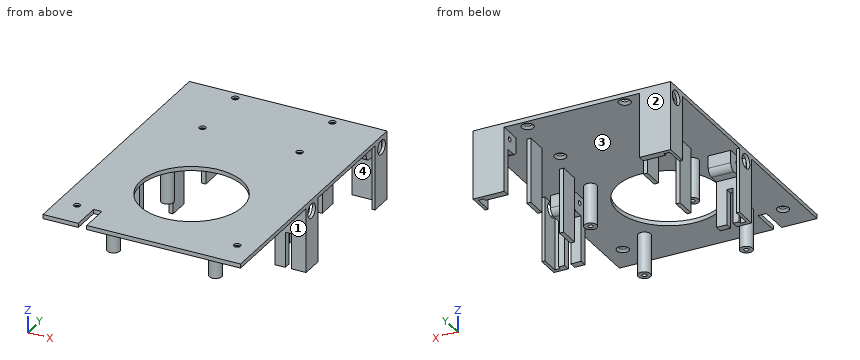
```python
from build123d import *

# Parameters (mm, degrees)
SKETCH1_W                                 = 95
SKETCH1_H                                 = 134
BOSS_EXTRUDE1_DEPTH                       = 2
CSK_FOR_4_FLAT_HEAD_MACHINE_SCREW_2_COUNT = 2
CSK_FOR_4_FLAT_HEAD_MACHINE_SCREW_2_PITCH = 46.7
CSK_FOR_4_FLAT_HEAD_MACHINE_SCREW_3_COUNT = 2
CSK_FOR_4_FLAT_HEAD_MACHINE_SCREW_3_PITCH = 55.505765466
CSK_FOR_4_FLAT_HEAD_MACHINE_SCREW_4_COUNT = 2
CSK_FOR_4_FLAT_HEAD_MACHINE_SCREW_4_PITCH = 30
CSK_FOR_4_FLAT_HEAD_MACHINE_SCREW_5_COUNT = 2
CSK_FOR_4_FLAT_HEAD_MACHINE_SCREW_5_PITCH = 116.985137945
CSK_FOR_4_FLAT_HEAD_MACHINE_SCREW_6_COUNT = 2
CSK_FOR_4_FLAT_HEAD_MACHINE_SCREW_6_PITCH = 131.458824352
SKETCH13_R                                = 24.6
CUT_EXTRUDE2_DEPTH                        = 165.271117364
SKETCH14_R                                = 3
BOSS_EXTRUDE4_DEPTH                       = 19.3
SKETCH15_R                                = 1.15
CUT_EXTRUDE3_DEPTH                        = 15
SKETCH16_W                                = 4
SKETCH16_H                                = 14
CUT_EXTRUDE4_DEPTH                        = 166.388905311
SKETCH17_W                                = 15
SKETCH17_H                                = 11
BOSS_EXTRUDE5_DEPTH                       = 31
SKETCH18_W                                = 2.7
SKETCH18_H                                = 70
CUT_EXTRUDE5_DEPTH                        = 31
SKETCH19_W                                = 14.3
SKETCH19_H                                = 67
CUT_EXTRUDE6_DEPTH                        = 22
FILLET5_R                                 = 3
FILLET6_R                                 = 3
FILLET7_R                                 = 3
FILLET8_R                                 = 3
SKETCH20_W                                = 2
SKETCH20_H                                = 10
BOSS_EXTRUDE6_DEPTH                       = 31
CUT_EXTRUDE7_DEPTH                        = 165.807888161
CUT_EXTRUDE7_DEPTH_BACK                   = 165.807888161
SKETCH22_R                                = 1.15
SKETCH23_R                                = 3.5
CUT_EXTRUDE8_DEPTH                        = 1.5
CUT_EXTRUDE9_START                        = -1.5
SKETCH24_R                                = 3.5
CUT_EXTRUDE9_DEPTH                        = 1.5
SKETCH25_W                                = 3
SKETCH25_H                                = 3.5
CUT_EXTRUDE10_DEPTH                       = 17


with BuildPart() as part:
    # Sketch1 → Boss-Extrude1 (new body)
    with BuildSketch(Plane.XY):
        with Locations((47.5, 67)):
            Rectangle(SKETCH1_W, SKETCH1_H)
    extrude(amount=BOSS_EXTRUDE1_DEPTH)

    # Sketch8 → CSK for #4 Flat Head Machine Screw (100)2 (revolve, cut)
    with BuildSketch(Plane(origin=(70.85, 130, 0), x_dir=(0, 1, 0), z_dir=(1, 0, 0))):
        Polygon((0, 0), (0, 2), (1.63195, 2), (1.63195, 1.028358553), (2.8575, 0), align=None)
    csk_for_4_flat_head_machine_screw_100 = revolve(axis=Axis((70.85, 130, -6.35), (0, 0, 1)), mode=Mode.SUBTRACT)

    # CSK for _4 Flat Head Machine Screw _ 2: CSK for #4 Flat Head Machine Screw (100)2 ×2
    with Locations(*[(-i * CSK_FOR_4_FLAT_HEAD_MACHINE_SCREW_2_PITCH, 0, 0) for i in range(1, CSK_FOR_4_FLAT_HEAD_MACHINE_SCREW_2_COUNT)]):
        add(csk_for_4_flat_head_machine_screw_100, mode=Mode.SUBTRACT)

    # CSK for _4 Flat Head Machine Screw _ 3: CSK for #4 Flat Head Machine Screw (100)2 ×2
    with Locations(*[Vector(-0.8413540396691381, -0.540484393791738, 0) * (i * CSK_FOR_4_FLAT_HEAD_MACHINE_SCREW_3_PITCH) for i in range(1, CSK_FOR_4_FLAT_HEAD_MACHINE_SCREW_3_COUNT)]):
        add(csk_for_4_flat_head_machine_screw_100, mode=Mode.SUBTRACT)

    # CSK for _4 Flat Head Machine Screw _ 4: CSK for #4 Flat Head Machine Screw (100)2 ×2
    with Locations(*[(0, -i * CSK_FOR_4_FLAT_HEAD_MACHINE_SCREW_4_PITCH, 0) for i in range(1, CSK_FOR_4_FLAT_HEAD_MACHINE_SCREW_4_COUNT)]):
        add(csk_for_4_flat_head_machine_screw_100, mode=Mode.SUBTRACT)

    # CSK for _4 Flat Head Machine Screw _ 5: CSK for #4 Flat Head Machine Screw (100)2 ×2
    with Locations(*[Vector(0.12950362982970207, -0.991578947870986, 0) * (i * CSK_FOR_4_FLAT_HEAD_MACHINE_SCREW_5_PITCH) for i in range(1, CSK_FOR_4_FLAT_HEAD_MACHINE_SCREW_5_COUNT)]):
        add(csk_for_4_flat_head_machine_screw_100, mode=Mode.SUBTRACT)

    # CSK for _4 Flat Head Machine Screw _ 6: CSK for #4 Flat Head Machine Screw (100)2 ×2
    with Locations(*[Vector(-0.47048952632046626, -0.8824055788710445, 0) * (i * CSK_FOR_4_FLAT_HEAD_MACHINE_SCREW_6_PITCH) for i in range(1, CSK_FOR_4_FLAT_HEAD_MACHINE_SCREW_6_COUNT)]):
        add(csk_for_4_flat_head_machine_screw_100, mode=Mode.SUBTRACT)

    # Sketch13 → Cut-Extrude2 (cut, through all)
    with BuildSketch(Plane(origin=(0, 0, 0), x_dir=(-1, 0, 0), z_dir=(0, 0, -1))):
        with Locations((-47.5, 45.5)):
            Circle(SKETCH13_R)
    extrude(amount=-CUT_EXTRUDE2_DEPTH, mode=Mode.SUBTRACT)

    # Sketch14 → Boss-Extrude4 (add)
    with BuildSketch(Plane(origin=(0, 0, 0), x_dir=(-1, 0, 0), z_dir=(0, 0, -1))):
        with Locations((-72, 70.1)):
            Circle(SKETCH14_R)
        with Locations((-23, 70.1)):
            Circle(SKETCH14_R)
        with Locations((-72, 20.9)):
            Circle(SKETCH14_R)
        with Locations((-23, 20.9)):
            Circle(SKETCH14_R)
    extrude(amount=BOSS_EXTRUDE4_DEPTH)

    # Sketch15 → Cut-Extrude3 (cut)
    with BuildSketch(Plane(origin=(0, 0, -19.3), x_dir=(-1, 0, 0), z_dir=(0, 0, -1))):
        with Locations((-72, 70.1)):
            Circle(SKETCH15_R)
        with Locations((-23, 70.1)):
            Circle(SKETCH15_R)
        with Locations((-23, 20.9)):
            Circle(SKETCH15_R)
        with Locations((-72, 20.9)):
            Circle(SKETCH15_R)
    extrude(amount=-CUT_EXTRUDE3_DEPTH, mode=Mode.SUBTRACT)

    # Sketch16 → Cut-Extrude4 (cut, through all)
    with BuildSketch(Plane(origin=(0, 0, 0), x_dir=(-1, 0, 0), z_dir=(0, 0, -1))):
        with Locations((-19, 7)):
            Rectangle(SKETCH16_W, SKETCH16_H)
    extrude(amount=-CUT_EXTRUDE4_DEPTH, mode=Mode.SUBTRACT)

    # Sketch17 → Boss-Extrude5 (add)
    with BuildSketch(Plane(origin=(0, 0, 0), x_dir=(-1, 0, 0), z_dir=(0, 0, -1))):
        with Locations((-87.5, 128.5)):
            Rectangle(SKETCH17_W, SKETCH17_H)
        with Locations((-87.5, 65.5)):
            Rectangle(SKETCH17_W, SKETCH17_H)
        with Locations((-7.5, 65.5)):
            Rectangle(SKETCH17_W, SKETCH17_H)
        with Locations((-7.5, 128.5)):
            Rectangle(SKETCH17_W, SKETCH17_H)
    extrude(amount=BOSS_EXTRUDE5_DEPTH)

    # Sketch18 → Cut-Extrude5 (cut)
    with BuildSketch(Plane(origin=(0, 0, -31), x_dir=(-1, 0, 0), z_dir=(0, 0, -1))):
        with Locations((-92.15, 97)):
            Rectangle(SKETCH18_W, SKETCH18_H)
        with Locations((-2.85, 97)):
            Rectangle(SKETCH18_W, SKETCH18_H)
    extrude(amount=-CUT_EXTRUDE5_DEPTH, mode=Mode.SUBTRACT)

    # Sketch19 → Cut-Extrude6 (cut)
    with BuildSketch(Plane(origin=(0, 0, -31), x_dir=(-1, 0, 0), z_dir=(0, 0, -1))):
        with Locations((-83.65, 97)):
            Rectangle(SKETCH19_W, SKETCH19_H)
        with Locations((-11.35, 97)):
            Rectangle(SKETCH19_W, SKETCH19_H)
    extrude(amount=-CUT_EXTRUDE6_DEPTH, mode=Mode.SUBTRACT)

    # Fillet5
    fillet5_edges = [part.edges().sort_by_distance(p)[0] for p in [
        (85.4, 123, -9),
    ]]
    fillet(fillet5_edges, radius=FILLET5_R)

    # Fillet6
    fillet6_edges = [part.edges().sort_by_distance(p)[0] for p in [
        (9.6, 123, -9),
    ]]
    fillet(fillet6_edges, radius=FILLET6_R)

    # Fillet7
    fillet7_edges = [part.edges().sort_by_distance(p)[0] for p in [
        (9.6, 71, -9),
    ]]
    fillet(fillet7_edges, radius=FILLET7_R)

    # Fillet8
    fillet8_edges = [part.edges().sort_by_distance(p)[0] for p in [
        (85.4, 71, -9),
    ]]
    fillet(fillet8_edges, radius=FILLET8_R)

    # Sketch20 → Boss-Extrude6 (add)
    with BuildSketch(Plane(origin=(0, 0, 0), x_dir=(-1, 0, 0), z_dir=(0, 0, -1))):
        with Locations((-75.5, 115)):
            Rectangle(SKETCH20_W, SKETCH20_H)
        with Locations((-75.5, 85)):
            Rectangle(SKETCH20_W, SKETCH20_H)
        with Locations((-19.5, 85)):
            Rectangle(SKETCH20_W, SKETCH20_H)
        with Locations((-19.5, 115)):
            Rectangle(SKETCH20_W, SKETCH20_H)
    extrude(amount=BOSS_EXTRUDE6_DEPTH)

    # Sketch22 → Cut-Extrude7 (cut, two sides: drawn at the far end of the back side and taken through both)
    with BuildSketch(Plane(origin=(90.8, 0, 0), x_dir=(0, 0, -1), z_dir=(1, 0, 0)).offset(-CUT_EXTRUDE7_DEPTH_BACK)):
        with Locations((3.5, 129)):
            Circle(SKETCH22_R)
        with Locations(Location((3.5, 65, 0), (0, 0, 90))):
            Circle(SKETCH22_R)
    extrude(amount=CUT_EXTRUDE7_DEPTH + CUT_EXTRUDE7_DEPTH_BACK, mode=Mode.SUBTRACT)

    # Sketch23 → Cut-Extrude8 (cut)
    with BuildSketch(Plane(origin=(95, 0, 0), x_dir=(0, 0, -1), z_dir=(1, 0, 0))):
        with Locations((3.5, 129)):
            Circle(SKETCH23_R)
        with Locations((3.5, 65)):
            Circle(SKETCH23_R)
    extrude(amount=-CUT_EXTRUDE8_DEPTH, mode=Mode.SUBTRACT)

    # Sketch24 → Cut-Extrude9 (cut)
    with BuildSketch(Plane.ZY.offset(CUT_EXTRUDE9_START)):
        with Locations(Location((-3.5, 129, 0), (0, 0, 180))):
            Circle(SKETCH24_R)
        with Locations(Location((-3.5, 65, 0), (0, 0, 180))):
            Circle(SKETCH24_R)
    extrude(amount=CUT_EXTRUDE9_DEPTH, mode=Mode.SUBTRACT)

    # Sketch25 → Cut-Extrude10 (cut)
    with BuildSketch(Plane(origin=(0, 0, -31), x_dir=(-1, 0, 0), z_dir=(0, 0, -1))):
        with Locations((-8.5, 61.75)):
            Rectangle(SKETCH25_W, SKETCH25_H)
        with Locations((-86.5, 61.75)):
            Rectangle(SKETCH25_W, SKETCH25_H)
    extrude(amount=-CUT_EXTRUDE10_DEPTH, mode=Mode.SUBTRACT)


solid = part.part
```
Part model, mm, in its own coordinate system. Face numbers are marked on the shaded views. Give positions to 0.01 mm unless a question says otherwise; leave off trailing zeros. Write each loop counter-clockwise with the first axis right and the second up, starting at its lowest first coordinate (ties: lowest second). Pieces come first, ordered by that corner, then holes. Notation, with made-up numbers: (-36, 69) -> (-16, 69) arc R23 cw to (-16, 100) -> close; hole circle Ø1 at (88, 5). An arc over 180 degrees is marked (long way). Put each result on its own line as item: value. Start each with the question number.
Item 1: Cut at B-B (x = 47.5). List the corners of the cut face in (y, z), then the cut area to 3 significant figures.
Item 2: Pin check, flat tips, straight feed: pin 1 Ø4 at (x, z) = (82, -17.5) entering from -Y; pin 2 Ø5 at (y, z) = (115, -22) entering from +X; pin 3 Ø5 at (y, z) = (114.5, -19) entering from -X; pin 4 Ø4.5 at (y, z) = (125.5, -12.5) entering from -X. Stop position of each tip, or through.
Item 3: Cut at C-C (y = 45.5). List the corners of the cut face in (x, z), then the cut area to 3 significant figures.
Item 4: Pull direction Y, two halves, no side cores. Call the marked faces 1, 2, 3 and 4: pulls with the +Y half, pulls with the -Y half, needs draft (parallel to the pull), parting line crosses it, or undercut.
Item 5: Cut at D-D (y = 86). List the corners of the cut face in (x, z).
Item 6: Wall check: L1, parallel to X at y = 130, z = 1.5; L2, parallel to Y at x = 94.2, z = -3.5; L3, parallel to Y at x = 23, z = -14. Give the ranges that are in metal, low to high. Write a range as [from, to].
Item 7: Cut at A-A (y = 100). List the corners of the cut face in (x, z).
Answer list:
1. outline: (0, 0) -> (20.9, 0) -> (20.9, 2) -> (0, 2) -> close; (70.1, 0) -> (134, 0) -> (134, 2) -> (70.1, 2) -> close
1. area: 170 mm2
2. pin 1: stops at y = 60
2. pin 2: stops at x = 76.5
2. pin 3: stops at x = 18.5
2. pin 4: stops at x = 0
3. outline: (0, 0) -> (22.9, 0) -> (22.9, 2) -> (0, 2) -> close; (72.1, 0) -> (95, 0) -> (95, 2) -> (72.1, 2) -> close
3. area: 91.6 mm2
4. face 1: pulls with the -Y half
4. face 2: pulls with the +Y half
4. face 3: undercut
4. face 4: undercut
5. outline: (0, 0) -> (18.5, 0) -> (18.5, -31) -> (20.5, -31) -> (20.5, 0) -> (74.5, 0) -> (74.5, -31) -> (76.5, -31) -> (76.5, 0) -> (95, 0) -> (95, 2) -> (0, 2) -> close
6. L1: x = [0, 22.52], [25.78, 69.22], [72.48, 95]
6. L2: y = [60, 61.5], [68.5, 71], [123, 125.5], [132.5, 134]
6. L3: y = [17.9, 19.75], [22.05, 23.9], [67.1, 68.95], [71.25, 73.1]
7. outline: (0, 0) -> (21.29, 0) -> (22.52, 1.03) -> (22.52, 2) -> (0, 2) -> close; (25.78, 1.03) -> (27.01, 0) -> (67.99, 0) -> (69.22, 1.03) -> (69.22, 2) -> (25.78, 2) -> close; (72.48, 1.03) -> (73.71, 0) -> (95, 0) -> (95, 2) -> (72.48, 2) -> close
